from build123d import *

# Parameters (mm, degrees)
SKETCH1_W           = 22.5
SKETCH1_H           = 11.8
BOSS_EXTRUDE1_DEPTH = 22.7
SKETCH2_W           = 4.7
SKETCH2_H           = 11.8
BOSS_EXTRUDE2_DEPTH = 2.5
BOSS_EXTRUDE3_DEPTH = 4
CUT_EXTRUDE1_DEPTH  = 2.5
SKETCH5_R           = 2.3
SKETCH5_R_2         = 0.85
BOSS_EXTRUDE4_DEPTH = 3.2


with BuildPart() as part:
    # Sketch1 → Boss-Extrude1 (new body)
    with BuildSketch(Plane(origin=(0, 0, 0), x_dir=(1, 0, 0), z_dir=(0, 1, 0))):
        with Locations((11.25, 5.9)):
            Rectangle(SKETCH1_W, SKETCH1_H)
    extrude(amount=BOSS_EXTRUDE1_DEPTH)

    # Sketch2 → Boss-Extrude2 (add)
    with BuildSketch(Plane(origin=(0, 15.89999995, 0), x_dir=(-1, 0, 0), z_dir=(0, -1, 0))):
        with Locations((-24.85, 5.9)):
            Rectangle(SKETCH2_W, SKETCH2_H)
        with Locations((2.35, 5.9)):
            Rectangle(SKETCH2_W, SKETCH2_H)
    extrude(amount=-BOSS_EXTRUDE2_DEPTH)

    # Sketch3 → Boss-Extrude3 (add)
    with BuildSketch(Plane(origin=(0, 22.7, 0), x_dir=(1, 0, 0), z_dir=(0, 1, 0))):
        with BuildLine():
            Line((12.2, 8.4), (11.244155686, 8.4))
            ThreePointArc((11.244155686, 8.4), (0, 5.9), (11.244155686, 3.4))
            Line((11.244155686, 3.4), (12.2, 3.4))
            ThreePointArc((12.2, 3.4), (14.7, 5.9), (12.2, 8.4))
        make_face()
    extrude(amount=BOSS_EXTRUDE3_DEPTH)

    # Sketch4 → Cut-Extrude1 (cut)
    with BuildSketch(Plane(origin=(0, 18.39999995, 0), x_dir=(1, 0, 0), z_dir=(0, 1, 0))):
        with BuildLine():
            Line((-4.7, 6.55), (-4.7, 5.25))
            Line((-4.7, 5.25), (-3.109934208, 5.25))
            ThreePointArc((-3.109934208, 5.25), (-1.35, 5.9), (-3.109934208, 6.55))
            Line((-3.109934208, 6.55), (-4.7, 6.55))
        make_face()
        with BuildLine():
            Line((27.2, 6.55), (27.2, 5.25))
            Line((27.2, 5.25), (25.609934208, 5.25))
            ThreePointArc((25.609934208, 5.25), (23.85, 5.9), (25.609934208, 6.55))
            Line((25.609934208, 6.55), (27.2, 6.55))
        make_face()
    extrude(amount=-CUT_EXTRUDE1_DEPTH, mode=Mode.SUBTRACT)

    # Sketch5 → Boss-Extrude4 (add)
    with BuildSketch(Plane(origin=(0, 26.7, 0), x_dir=(1, 0, 0), z_dir=(0, 1, 0))):
        with Locations((5.9, 5.9)):
            Circle(SKETCH5_R)
        with Locations((5.9, 5.9)):
            Circle(SKETCH5_R_2, mode=Mode.SUBTRACT)
    extrude(amount=BOSS_EXTRUDE4_DEPTH)


solid = part.part
Could you check a few things on this model? Use its own coordinates, in mm. A direction names the side the tool comes from. Coordinates: 2 decimals unless noted, no trailing zeros. Order: outer loops, then holes, each group sorted by start corner. A loop starts at its lowest first (then second) coordinate and runs counter-clockwise, first axis right, second up.
Q1. Will these pins go through, and if not, where does the flat tip stop? pin 1 (3 mm diameter, centred on y = 5.5, z = -1.5, fed in from +X); pin 2 (5 mm diameter, centred on y = 25.5, z = -4, fed in from +X); pin 3 (2 mm diameter, centred on x = 18.5, z = -9.5, fed in from +Y); pin 4 (1.9 mm diameter, centred on x = 6.5, z = -6, fed in from +Y).
Q2. Which directions (+Z, -Z, +X, -X, +Y, -Y) give clear straight access to the entire face, cutting with the end or side of a thin tool? Please do faces 1 (the flat face through (24.9, 15.9, -7.3)), 2 (the flat face through (16, 22.7, -6)), 3 (the flat face through (-1, 18.4, -6)).
Q3. Suppose I cut it at C-C on y = 23.25. Please give me the cut outline in (x, z).
Q4. Suppose I cut it at A-A on x = 24.85. Please give me the cut outline in (y, z), and give its area (3 significant figures).
Q5. Please list where these lines run through material, in increasing order: L1, parallel to X at y = 16.6, z = -5.9; L2, parallel to Y at x = 22, z = -4.75; L3, parallel to Y at x = 8, z = -3.75.
Q6. Suppose I cut it at B-B on z = -1. Please give me the cut outline in (x, y).
Q7. Suppose I cut it at D-D on x = 18. Please give me the cut outline in (y, z), and give its area (3 significant figures).
Q8. Thinking about a two-plate mould opening in X: for faces 4 (the cylindrical face through (5.789, 28.278, -6.743)), 5 (the flat face through (22.5, 21, -6)), 6 (the flat face through (12, 25, -3.4)), 7 (the flat face through (6, 26.7, -6)), which applies, released by +X, released by -X, zero draft, split by the parting line, or undercut?
Answer:
1. pin 1: stops at x = 22.5
1. pin 2: stops at x = 14.7
1. pin 3: stops at y = 22.7
1. pin 4: stops at y = 29.9
2. face 1: +Z, -Z, +X, -Y
2. face 2: +X, +Y
2. face 3: +Z, -Z, -X, +Y
3. outline: (11.24, -8.4) - (12.2, -8.4) arc R2.5 ccw to (12.2, -3.4) - (11.24, -3.4) arc R5.9 ccw (long way) to start
4. outline: (15.9, -11.8) - (18.4, -11.8) - (18.4, -6.9) - (15.9, -6.9) - close; (15.9, -4.9) - (18.4, -4.9) - (18.4, 0) - (15.9, 0) - close
4. area: 24.5 mm2
5. L1: x = -1.35 to 23.85
5. L2: y = 0 to 22.7
5. L3: y = 0 to 26.7
6. outline: (-4.7, 15.9) - (0, 15.9) - (0, 0) - (22.5, 0) - (22.5, 15.9) - (27.2, 15.9) - (27.2, 18.4) - (22.5, 18.4) - (22.5, 22.7) - (9.19, 22.7) - (9.19, 26.7) - (2.61, 26.7) - (2.61, 22.7) - (0, 22.7) - (0, 18.4) - (-4.7, 18.4) - close
7. outline: (0, -11.8) - (22.7, -11.8) - (22.7, 0) - (0, 0) - close
7. area: 268 mm2
8. face 4: undercut
8. face 5: released by +X
8. face 6: zero draft
8. face 7: undercut
